```python
from build123d import *

# Parameters (mm, degrees)
SKETCH013_W   = 17.7
SKETCH013_H   = 25
SKETCH013_W_2 = 14.7
SKETCH013_H_2 = 22
PAD001_DEPTH  = 9.75
SKETCH014_W   = 1.35
SKETCH014_H   = 1.5
SKETCH014_W_2 = 4.25
PAD002_DEPTH  = 14.7
CHAMFER_SIZE  = 1


with BuildPart() as part:
    # Sketch013 → Pad001 (new body)
    with BuildSketch(Plane.XY):
        Rectangle(SKETCH013_W, SKETCH013_H)
        Rectangle(SKETCH013_W_2, SKETCH013_H_2, mode=Mode.SUBTRACT)
    extrude(amount=PAD001_DEPTH)

    # Sketch014 (on Face7 of Pad001) → Pad002 (join)
    with BuildSketch(Plane.YZ.offset(-7.35)):
        with Locations((-10.325, 0.75)):
            Rectangle(SKETCH014_W, SKETCH014_H)
        with Locations((-10.325, 9)):
            Rectangle(SKETCH014_W, SKETCH014_H)
        with Locations((10.325, 9)):
            Rectangle(SKETCH014_W, SKETCH014_H)
        with Locations((8.875, 0.75)):
            Rectangle(SKETCH014_W_2, SKETCH014_H)
    extrude(amount=PAD002_DEPTH)

    # Chamfer
    chamfer_edges = [part.edges().sort_by_distance(p)[0] for p in [
        (0, -9.65, 9.75),
        (0, 9.65, 9.75),
        (0, 6.75, 1.5),
    ]]
    chamfer(chamfer_edges, length=CHAMFER_SIZE)


solid = part.part
```
Check sheet for the modelled part. Datum: model origin and axes. Units: mm. A direction names the side the tool comes from. Give positions to 0.01 mm unless a question says otherwise; leave off trailing zeros. Write each loop counter-clockwise with the first axis right and the second up, starting at its lowest first coordinate (ties: lowest second). Pieces come first, ordered by that corner, then holes. Notation, with made-up numbers: (81.25, -15) -> (135.25, -15) arc R23 ccw to (135.25, 18) -> close; hole circle Ø2 at (40, 76). An arc over 180 degrees is marked (long way). Use CSV: the item, a comma, the result in double quotes. Start each with the question number.
Q1. Scan lines: line 1 along Y through (x, z) = (-4.25, 5.5); line 2 along X through (y, z) = (-2, 1.25); line 3 along Y through (x, z) = (-4, 9.5). Record each from-to range of solid material in increasing order.
Q2. Cross-section at D-D on y = -10.25. Enter the section's corners in (x, z).
Q3. Cross-section at B-B on z = 2. Enter the section's corners in (x, y).
Q4. Release check for a two-part mould opening along Z. For faces 5 (the flat face through (-0.1, 7.26, 1.01)), 6 (the flat face through (8.85, 0, 5)), 7 (the flat face through (0, -10, 8.25)) record: +Z half, -Z half, draft (parallel to the pull), parting line (faces both ways), or undercut.
Q5. Cross-section at C-C on x = 2.5. Enter the section's corners in (y, z).
Q6. Cross-section at A-A on y = -7. Enter the section's corners in (x, z), and give its area (4 significant figures).
Q7. Depth check by flat-ended pin: P1, Ø1.1, axis at x = -3, y = -10, coming from the +Z side. Enter the tip coordinate at first touch or a pass-through.
Q8. Tool access check on faces 1 (the flat face through (0, -9.65, 1)), 2 (the flat face through (-8.85, 0, 5)), 3 (the flat face through (0, -11, 5)), 4 (the flat face through (-0.1, -10.1, 9.2)). Record the directions out of +Z, -Z, +X, -X, +Y, -Y that give a thin tool (end or side, any length) a straight path to the whole face; none if there is none.
Working result:
1,line 1,"y = -12.5 to -11, 11 to 12.5"
1,line 2,"x = -8.85 to -7.35, 7.35 to 8.85"
1,line 3,"y = -12.5 to -10.4, 10.4 to 12.5"
2,outline,"(-8.85, 0) -> (8.85, 0) -> (8.85, 9.75) -> (7.35, 9.75) -> (7.35, 9.35) -> (-7.35, 9.35) -> (-7.35, 9.75) -> (-8.85, 9.75) -> close; hole (-7.35, 1.5) -> (7.35, 1.5) -> (7.35, 8.25) -> (-7.35, 8.25) -> close"
3,outline,"(-8.85, -12.5) -> (8.85, -12.5) -> (8.85, 12.5) -> (-8.85, 12.5) -> close; hole (-7.35, -11) -> (7.35, -11) -> (7.35, 11) -> (-7.35, 11) -> close"
4,face 5,"+Z half"
4,face 6,"draft"
4,face 7,"undercut"
5,outline,"(-12.5, 0) -> (-9.65, 0) -> (-9.65, 1.5) -> (-11, 1.5) -> (-11, 8.25) -> (-9.65, 8.25) -> (-9.65, 8.75) -> (-10.65, 9.75) -> (-12.5, 9.75) -> close; (6.75, 0) -> (12.5, 0) -> (12.5, 9.75) -> (10.65, 9.75) -> (9.65, 8.75) -> (9.65, 8.25) -> (11, 8.25) -> (11, 1.5) -> (7.75, 1.5) -> (6.75, 0.5) -> close"
6,outline,"(-8.85, 0) -> (-7.35, 0) -> (-7.35, 9.75) -> (-8.85, 9.75) -> close; (7.35, 0) -> (8.85, 0) -> (8.85, 9.75) -> (7.35, 9.75) -> close"
6,area,"29.25 mm^2"
7,P1,"stops at z = 9.65"
8,face 1,"+Z, -Z"
8,face 2,"+Z, -Z, -X, +Y, -Y"
8,face 3,"none"
8,face 4,"+Z"
